from build123d import *

# Parameters (mm, degrees)
CROQUIS8_R              = 1.5
CROQUIS8_W              = 60
CROQUIS8_H              = 60
SALIENTE_EXTRUIR1_DEPTH = 3
CROQUIS14_R             = 1.5
CORTAR_EXTRUIR5_DEPTH   = 162.582796114
CROQUIS15_R             = 1.5
CORTAR_EXTRUIR6_DEPTH   = 162.582796114
CORTAR_EXTRUIR7_DEPTH   = 23
CROQUIS17_R             = 1.5
CROQUIS17_R_2           = 1.55
CORTAR_EXTRUIR8_DEPTH   = 10
CROQUIS18_R             = 1.2
CORTAR_EXTRUIR9_DEPTH   = 10
CROQUIS19_R             = 1.5
CORTAR_EXTRUIR10_DEPTH  = 10
CROQUIS20_R             = 1.5
CORTAR_EXTRUIR11_DEPTH  = 10
CORTAR_EXTRUIR12_DEPTH  = 10


with BuildPart() as part:
    # Croquis8 → Saliente-Extruir1 (new body)
    with BuildSketch(Plane.XY):
        with BuildLine():
            Line((-30, -150), (30, -150))
            ThreePointArc((30, -150), (37.071067812, -147.071067812), (40, -140))
            Line((40, -140), (40, -74.142135624))
            ThreePointArc((40, -74.142135624), (40.761204675, -70.3153013), (42.928932188, -67.071067812))
            Line((42.928932188, -67.071067812), (57.071067812, -52.928932188))
            ThreePointArc((57.071067812, -52.928932188), (59.238795325, -49.6846987), (60, -45.857864376))
            Line((60, -45.857864376), (60, 140))
            ThreePointArc((60, 140), (57.071067812, 147.071067812), (50, 150))
            Line((50, 150), (-50, 150))
            ThreePointArc((-50, 150), (-57.071067812, 147.071067812), (-60, 140))
            Line((-60, 140), (-60, -45.857864376))
            ThreePointArc((-60, -45.857864376), (-59.238795325, -49.6846987), (-57.071067812, -52.928932188))
            Line((-57.071067812, -52.928932188), (-42.928932188, -67.071067812))
            ThreePointArc((-42.928932188, -67.071067812), (-40.761204675, -70.3153013), (-40, -74.142135624))
            Line((-40, -74.142135624), (-40, -140))
            ThreePointArc((-40, -140), (-37.071067812, -147.071067812), (-30, -150))
        make_face()
        with Locations((33.6, 66.5)):
            Circle(CROQUIS8_R, mode=Mode.SUBTRACT)
        with Locations((56.4, 66.5)):
            Circle(CROQUIS8_R, mode=Mode.SUBTRACT)
        with Locations((56.4, 93.5)):
            Circle(CROQUIS8_R, mode=Mode.SUBTRACT)
        with Locations((33.6, 93.5)):
            Circle(CROQUIS8_R, mode=Mode.SUBTRACT)
        with Locations((13.5, 40)):
            Circle(CROQUIS8_R, mode=Mode.SUBTRACT)
        with Locations((13.5, 20)):
            Circle(CROQUIS8_R, mode=Mode.SUBTRACT)
        with Locations((-13.5, 20)):
            Circle(CROQUIS8_R, mode=Mode.SUBTRACT)
        with Locations((-13.5, 40)):
            Circle(CROQUIS8_R, mode=Mode.SUBTRACT)
        with Locations((-56.4, 66.5)):
            Circle(CROQUIS8_R, mode=Mode.SUBTRACT)
        with Locations((-33.6, 66.5)):
            Circle(CROQUIS8_R, mode=Mode.SUBTRACT)
        with Locations((-33.6, 93.5)):
            Circle(CROQUIS8_R, mode=Mode.SUBTRACT)
        with Locations((-56.4, 93.5)):
            Circle(CROQUIS8_R, mode=Mode.SUBTRACT)
        with Locations((0, 80)):
            Rectangle(CROQUIS8_W, CROQUIS8_H, mode=Mode.SUBTRACT)
    extrude(amount=SALIENTE_EXTRUIR1_DEPTH)

    # Croquis14 → Cortar-Extruir5 (cut, through all)
    with BuildSketch(Plane(origin=(0, 0, 0), x_dir=(-1, 0, 0), z_dir=(0, 0, -1))):
        with Locations(Location((45, 135, 0), (0, 0, 180))):
            Circle(CROQUIS14_R)
        with Locations((-45, 135)):
            Circle(CROQUIS14_R)
        with Locations((-45, -45.857864376)):
            Circle(CROQUIS14_R)
        with Locations(Location((45, -45.857864376, 0), (0, 0, 180))):
            Circle(CROQUIS14_R)
        with Locations((45, 30)):
            Circle(CROQUIS14_R)
        with Locations(Location((-45, 30, 0), (0, 0, 180))):
            Circle(CROQUIS14_R)
    extrude(amount=-CORTAR_EXTRUIR5_DEPTH, mode=Mode.SUBTRACT)

    # Croquis15 → Cortar-Extruir6 (cut, through all)
    with BuildSketch(Plane(origin=(0, 0, 0), x_dir=(-1, 0, 0), z_dir=(0, 0, -1))):
        with Locations((30, 145)):
            Circle(CROQUIS15_R)
        with Locations(Location((-30, 145, 0), (0, 0, 180))):
            Circle(CROQUIS15_R)
        with Locations((20, -145)):
            Circle(CROQUIS15_R)
        with Locations(Location((-20, -145, 0), (0, 0, 180))):
            Circle(CROQUIS15_R)
        with Locations((55, -7.928932188)):
            Circle(CROQUIS15_R)
        with Locations(Location((-55, -7.928932188, 0), (0, 0, 180))):
            Circle(CROQUIS15_R)
    extrude(amount=-CORTAR_EXTRUIR6_DEPTH, mode=Mode.SUBTRACT)

    # Croquis16 → Cortar-Extruir7 (cut)
    with BuildSketch(Plane.XY.offset(3)):
        with BuildLine():
            Line((20.25, -64.5), (20.25, -55.5))
            Line((20.25, -55.5), (20.25, -54.5))
            Line((20.25, -54.5), (20.25, -45.5))
            ThreePointArc((20.25, -45.5), (20.103553391, -45.146446609), (19.75, -45))
            Line((19.75, -45), (-19.75, -45))
            ThreePointArc((-19.75, -45), (-20.103553391, -45.146446609), (-20.25, -45.5))
            Line((-20.25, -45.5), (-20.25, -54.5))
            Line((-20.25, -54.5), (-20.25, -55.5))
            Line((-20.25, -55.5), (-20.25, -64.5))
            ThreePointArc((-20.25, -64.5), (-20.103553391, -64.853553391), (-19.75, -65))
            Line((-19.75, -65), (19.75, -65))
            ThreePointArc((19.75, -65), (20.103553391, -64.853553391), (20.25, -64.5))
        make_face()
    extrude(amount=-CORTAR_EXTRUIR7_DEPTH, mode=Mode.SUBTRACT)

    # Croquis17 → Cortar-Extruir8 (cut)
    with BuildSketch(Plane(origin=(0, 0, 0), x_dir=(-1, 0, 0), z_dir=(0, 0, -1))):
        with Locations((-25, -113)):
            Circle(CROQUIS17_R)
        with Locations((25, -113)):
            Circle(CROQUIS17_R)
        with Locations((-18.5, -70.5)):
            Circle(CROQUIS17_R_2)
        with Locations((18.5, -70.5)):
            Circle(CROQUIS17_R_2)
        with Locations((-18.5, -103.5)):
            Circle(CROQUIS17_R_2)
        with Locations((18.5, -103.5)):
            Circle(CROQUIS17_R_2)
        with BuildLine():
            ThreePointArc((-6.75, -25), (-10.25, -21.5), (-13.75, -25))
            ThreePointArc((-13.75, -25), (-10.25, -28.5), (-6.75, -25))
        make_face()
    extrude(amount=-CORTAR_EXTRUIR8_DEPTH, mode=Mode.SUBTRACT)

    # Croquis18 → Cortar-Extruir9 (cut)
    with BuildSketch(Plane.XY.offset(3)):
        with Locations((1.6, -33.2)):
            Circle(CROQUIS18_R)
        with Locations((15.6, -33.2)):
            Circle(CROQUIS18_R)
    extrude(amount=-CORTAR_EXTRUIR9_DEPTH, mode=Mode.SUBTRACT)

    # Croquis19 → Cortar-Extruir10 (cut)
    with BuildSketch(Plane.XY.offset(3)):
        with Locations((-4, -135.549922457)):
            Circle(CROQUIS19_R)
        with Locations((4.000000635, -135.549923318)):
            Circle(CROQUIS19_R)
    extrude(amount=-CORTAR_EXTRUIR10_DEPTH, mode=Mode.SUBTRACT)

    # Croquis20 → Cortar-Extruir11 (cut)
    with BuildSketch(Plane.XY.offset(3)):
        with Locations((-30, 41.5)):
            Circle(CROQUIS20_R)
        with Locations((30, 41.5)):
            Circle(CROQUIS20_R)
    extrude(amount=-CORTAR_EXTRUIR11_DEPTH, mode=Mode.SUBTRACT)

    # Croquis22 → Cortar-Extruir12 (cut)
    with BuildSketch(Plane.XY.offset(3)):
        with BuildLine():
            ThreePointArc((26.312169292, -48.918229167), (22.4, -50.15), (26.312169292, -51.381770833))
            ThreePointArc((26.312169292, -51.381770833), (26.7, -50.15), (26.312169292, -48.918229167))
        make_face()
        with BuildLine():
            ThreePointArc((26.312169292, -58.618229167), (22.4, -59.85), (26.312169292, -61.081770833))
            ThreePointArc((26.312169292, -61.081770833), (26.7, -59.85), (26.312169292, -58.618229167))
        make_face()
        with BuildLine():
            ThreePointArc((-26.312169292, -61.081770833), (-22.4, -59.85), (-26.312169292, -58.618229167))
            ThreePointArc((-26.312169292, -58.618229167), (-26.7, -59.85), (-26.312169292, -61.081770833))
        make_face()
        with BuildLine():
            ThreePointArc((-26.312169292, -51.381770833), (-22.4, -50.15), (-26.312169292, -48.918229167))
            ThreePointArc((-26.312169292, -48.918229167), (-26.7, -50.15), (-26.312169292, -51.381770833))
        make_face()
    extrude(amount=-CORTAR_EXTRUIR12_DEPTH, mode=Mode.SUBTRACT)


solid = part.part
Source: CAD feature listing. Evaluate the final solid. Frame: model axes, mm. Round coordinates to 2 decimals unless told otherwise and drop trailing zeros. Order: outer loops, then holes, each group sorted by start corner. A loop starts at its lowest first (then second) coordinate and runs counter-clockwise, first axis right, second up. Notation, with made-up numbers: (32, 64) - (73, 64) arc R16 cw to (73, 93) - close; hole circle Ø5 at (87, 47). An arc over 180 degrees is marked (long way). Use a Markdown table: item, result. Add a question column.
1. Line query: probe 1 along Y at (x, z) = (25, 1.6); probe 2 along X at (y, z) = (135, 1.65); probe 3 along Y at (x, z) = (-1.5, 2.15). Output: solid intervals per line, ascending.
2. Mould query, pull axis X, two halves, no side actions, for faces 1 (the cylindrical face through (7.7, -27.4, 1.5)), 2 (the cylindrical face through (-37.15, -146.99, 1.48)), 3 (the cylindrical face through (57.15, 146.99, 1.48)). Classes: +X half, -X half, draft (parallel to the pull), parting line (faces both ways), or undercut.
3. Section query B-B (z = 2.55). Give the number of separate pieces and of enclosed holes in the cut face, then the cut area to 3 significant figures.
4. First-contact query: pin 1 (1.5 mm diameter, centred on y = -57, z = 2, fed in from -X); pin 2 (1.5 mm diameter, centred on x = -34.5, z = 2, fed in from -Y). Flat tips, straight axial feed; report the tip coordinate or a pass-through.
5. Section query A-A (y = -83). Return the cut outline in (x, z), then the cut area to 3 significant figures.
Derived:
| question | item | result |
|---|---|---|
| 1 | probe 1 | -150 to -114.5, -111.5 to -61.95, -57.75 to -52.25, -48.05 to 50, 110 to 150 |
| 1 | probe 2 | -60 to -46.5, -43.5 to 43.5, 46.5 to 60 |
| 1 | probe 3 | -150 to -65, -45 to 50, 110 to 150 |
| 2 | face 1 | undercut |
| 2 | face 2 | -X half |
| 2 | face 3 | +X half |
| 3 | separate pieces | 1 |
| 3 | enclosed holes | 43 |
| 3 | area | 27,600 mm2 |
| 4 | pin 1 | x = -53.75 |
| 4 | pin 2 | y = -149.27 |
| 5 | outline | (-40, 0) - (40, 0) - (40, 3) - (-40, 3) - close |
| 5 | area | 240 mm2 |
